from build123d import *

# Parameters (mm, degrees)
SKETCH_1_R               = 200
SKETCH_1_R_2             = 6.1
EXTRUDE_1_DEPTH          = 10
SKETCH_2_R               = 6.1
CUT_EXTRUDE_1_DEPTH      = 10
PATTERN_CIRCULAR_1_COUNT = 3
SKETCH_3_R               = 2.75
CUT_EXTRUDE_2_DEPTH      = 10
PATTERN_CIRCULAR_2_COUNT = 6


with BuildPart() as part:
    # Эскиз1 → Бобышка-Вытянуть1 (new body)
    with BuildSketch(Plane(origin=(0, 0, 0), x_dir=(1, 0, 0), z_dir=(0, 1, 0))):
        with Locations(Location((0, 0, 0), (0, 0, 270))):
            Circle(SKETCH_1_R)
        with Locations(Location((0, 0, 0), (0, 0, 270))):
            Circle(SKETCH_1_R_2, mode=Mode.SUBTRACT)
    extrude(amount=EXTRUDE_1_DEPTH)

    # Эскиз2 → Вырез-Вытянуть1 (cut)
    with BuildSketch(Plane(origin=(0, 10, 0), x_dir=(1, 0, 0), z_dir=(0, 1, 0))):
        with Locations(Location((-188, 0, 0), (0, 0, 270))):
            Circle(SKETCH_2_R)
    cut_extrude_1 = extrude(amount=-CUT_EXTRUDE_1_DEPTH, mode=Mode.SUBTRACT)

    # Круговой массив1: Вырез-Вытянуть1 ×3 about axis
    pattern_circular_1_axis = Axis((0, 0, 0), (0, 1, 0))
    for i in range(1, PATTERN_CIRCULAR_1_COUNT):
        add(cut_extrude_1.rotate(pattern_circular_1_axis, i * 360 / PATTERN_CIRCULAR_1_COUNT), mode=Mode.SUBTRACT)

    # Эскиз3 → Вырез-Вытянуть2 (cut)
    with BuildSketch(Plane(origin=(0, 10, 0), x_dir=(1, 0, 0), z_dir=(0, 1, 0))):
        with Locations(Location((-165.5, 0, 0), (0, 0, 270))):
            Circle(SKETCH_3_R)
    cut_extrude_2 = extrude(amount=-CUT_EXTRUDE_2_DEPTH, mode=Mode.SUBTRACT)

    # Круговой массив2: Вырез-Вытянуть2 ×6 about axis
    pattern_circular_2_axis = Axis((0, 0, 0), (0, 1, 0))
    for i in range(1, PATTERN_CIRCULAR_2_COUNT):
        add(cut_extrude_2.rotate(pattern_circular_2_axis, i * 360 / PATTERN_CIRCULAR_2_COUNT), mode=Mode.SUBTRACT)


solid = part.part
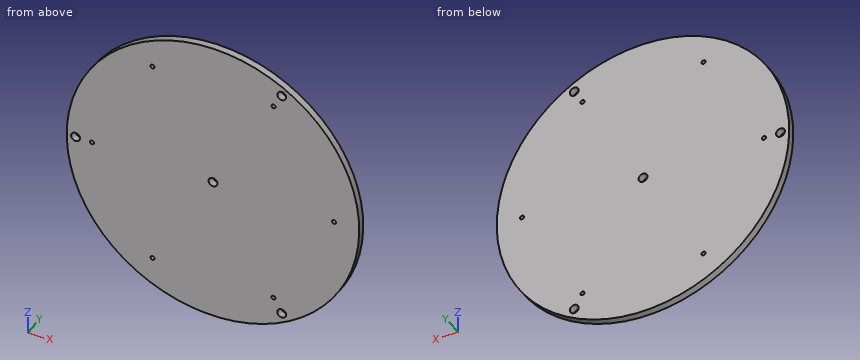
Geometry: final body of the model. Coordinates: model frame, mm. Coordinates: 2 decimals unless noted, no trailing zeros. Write each loop counter-clockwise with the first axis right and the second up, starting at its lowest first coordinate (ties: lowest second). Pieces come first, ordered by that corner, then holes. Notation, with made-up numbers: (-20, 8.5) - (-2, 8.5) arc R12 ccw to (-2, 21.5) - close; hole circle Ø8 at (-14.75, 23). An arc over 180 degrees is marked (long way). Return JSON: item names as keys, results as strings.
Item 1: Section query A-A (x = 0). Output: boundary loops of the cut face in (y, z), and give its area (3 significant figures).
Completed:
{"outline": "(0, -200) - (10, -200) - (10, -6.1) - (0, -6.1) - close; (0, 6.1) - (10, 6.1) - (10, 200) - (0, 200) - close", "area": "3,880 mm2"}
Item 2: Line query: L1, parallel to X at y = 1.75, z = -5; L2, parallel to Z at x = 5.5, y = 8.75; L3, parallel to Z at x = -165.5, y = 5.75. Output: solid intervals per line, ascending.
Completed:
{"L1": "x = -199.94 to -191.49, -184.51 to -3.49, 3.49 to 199.94", "L2": "z = -199.92 to -2.64, 2.64 to 199.92", "L3": "z = -112.29 to -2.75, 2.75 to 112.29"}
Item 3: Section query B-B (x = 94). Output: boundary loops of the cut face in (y, z), and give its area (3 significant figures).
Completed:
{"outline": "(0, -176.53) - (10, -176.53) - (10, -168.91) - (0, -168.91) - close; (0, -156.71) - (10, -156.71) - (10, 156.71) - (0, 156.71) - close; (0, 168.91) - (10, 168.91) - (10, 176.53) - (0, 176.53) - close", "area": "3,290 mm2"}
Item 4: Pin query (flat end, axial travel): pin 1 Ø2 at (y, z) = (8, 156) entering from +X; pin 2 Ø10 at (x, z) = (94, -162.81) entering from +Y (3 decimals); pin 3 Ø2 at (y, z) = (8.5, 132.5) entering from +X. Return the tip coordinate at first contact, or that it passes through.
Completed:
{"pin 1": "stops at x = 126.39", "pin 2": "passes through", "pin 3": "stops at x = 150.69"}
Item 5: Section query D-D (x = -188). Output: boundary loops of the cut face in (y, z), and give its area (3 significant figures).
Completed:
{"outline": "(0, -68.23) - (10, -68.23) - (10, -6.1) - (0, -6.1) - close; (0, 6.1) - (10, 6.1) - (10, 68.23) - (0, 68.23) - close", "area": "1,240 mm2"}
Item 6: Section query C-C (y = 6). Count the separate pieces of the cut face and the enclosed holes in it, and give its area (3 significant figures).
Completed:
{"separate pieces": "1", "enclosed holes": "10", "area": "125,000 mm2"}
